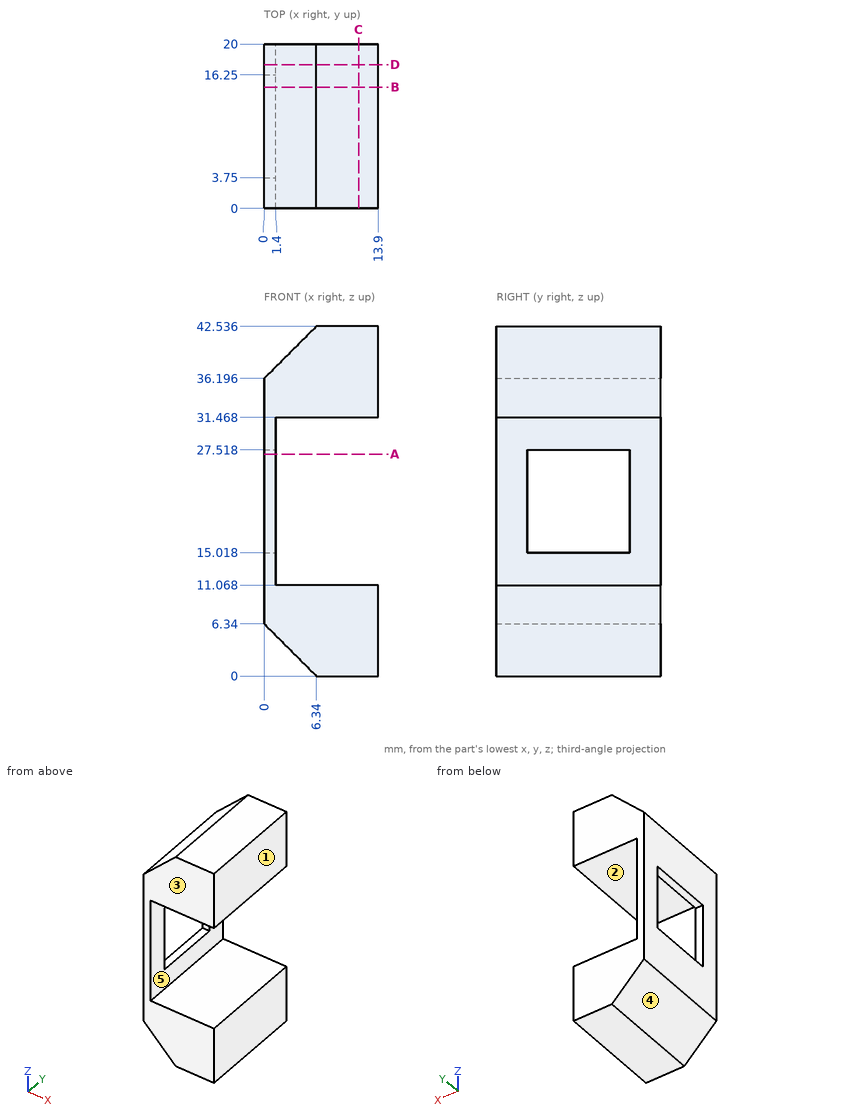
Geometry check sheet. Reference: drawing and pictorial views, mm from the part's lowest x, y, z. A direction names the side the tool comes from. Coordinates: 2 decimals unless noted, no trailing zeros. Order: outer loops, then holes, each group sorted by start corner. A loop starts at its lowest first (then second) coordinate and runs counter-clockwise, first axis right, second up. Notation, with made-up numbers: M 0,59.5 L 4,59.5 A23 ccw 4,73.5 Z; hole C 11.5,30.25 d5. An arc over 180 degrees is marked long. Write each question's results on one line, items separated by ' | '. Start each with the question number.
1. Cross-section at D-D on y = 17.5. Record the cut outline in (x, z).
2. Mould release check, pull along Z, two halves, no side actions. Record for the marked faces 3, 4 and 5: +Z half, -Z half, draft (parallel to the pull), parting line (faces both ways), or undercut.
3. Go/stop test with flat-tipped pins: P1, Ø3, axis at x = 10.5, y = 7, coming from the -Z side; P2, Ø1.5, axis at x = 1, y = 12.5, coming from the -Z side; P3, Ø1, axis at x = 5, y = 3, coming from the -Z side. Record where each tip stops, or that it passes through.
4. Cross-section at A-A on z = 27. Record the cut outline in (x, y).
5. Cross-section at B-B on y = 14.75. Record the cut outline in (x, z), and give its area (3 significant figures).
6. Access from +Z, -Z, +X, -X, +Y, -Y to the whole of each face (thin tool, end or side, straight path). Record for the marked faces 1 and 2.
7. Material ranges on probe 1 along Z at (x, y) = (13.25, 15.75); probe 2 along Z at (x, y) = (5.25, 18.75) (1 decimal); probe 3 along X at (y, z) = (12.5, 4), recorded low to high.
8. Cross-section at C-C on x = 11.5. Record the cut outline in (y, z), and give its area (3 significant figures).
Checks:
1) outline: M 0,6.34 L 6.34,0 L 13.9,0 L 13.9,11.07 L 1.4,11.07 L 1.4,31.47 L 13.9,31.47 L 13.9,42.54 L 6.34,42.54 L 0,36.2 Z
2) face 3: draft | face 4: -Z half | face 5: undercut
3) P1: stops at z = 0 | P2: stops at z = 4.59 | P3: stops at z = 0.84
4) outline: M 0,0 L 1.4,0 L 1.4,3.75 L 0,3.75 Z; M 0,16.25 L 1.4,16.25 L 1.4,20 L 0,20 Z
5) outline: M 0,6.34 L 6.34,0 L 13.9,0 L 13.9,11.07 L 1.4,11.07 L 1.4,15.02 L 0,15.02 Z; M 0,27.52 L 1.4,27.52 L 1.4,31.47 L 13.9,31.47 L 13.9,42.54 L 6.34,42.54 L 0,36.2 Z | area: 279 mm²
6) face 1: +Z, -Z, +X, +Y, -Y | face 2: +X, +Y, -Y
7) probe 1: z = 0 to 11.07, 31.47 to 42.54 | probe 2: z = 1.1 to 11.1, 31.5 to 41.4 | probe 3: x = 2.34 to 13.9
8) outline: M 0,0 L 20,0 L 20,11.07 L 0,11.07 Z; M 0,31.47 L 20,31.47 L 20,42.54 L 0,42.54 Z | area: 443 mm²
